The model under review builds one solid part; all positions refer to its coordinate system, in mm. A direction names the side the tool comes from. Round coordinates to 2 decimals unless told otherwise and drop trailing zeros. Order: outer loops, then holes, each group sorted by start corner. A loop starts at its lowest first (then second) coordinate and runs counter-clockwise, first axis right, second up.
1) Clearance check with flat-ended pins moving along their axes: P1, Ø8, axis at x = -67, z = -3.5, coming from the -Y side; P2, Ø1.5, axis at x = -6, z = -21.5, coming from the +Y side; P3, Ø9, axis at y = 243, z = -5.5, coming from the +X side; P4, Ø8, axis at x = 0, y = 260, coming from the +Z side. State where each tip first meets the part, or that it passes through.
2) To check wall thickness, follow L1, parallel to X at y = 260, z = -0.5; L2, parallel to X at y = 53, z = 0; L3, parallel to Y at x = 0, z = -8. State the ranges of each line that lie inside material, in increasing order.
3) Consider section C-C (x = 18). Give the boundary of the cut face in (y, z).
4) Consider section B-B (z = 0). Give the boundary of the cut face in (x, y), then the cut area to 3 significant figures.
5) Machinability: for faces 1 (the face through (10.382, 101.4, 19.961)), 2 (the face through (15, 245, 0)), 3 (the face through (-50, 100, 0)), which of the approach directions +Z, -Z, +X, -X, +Y, -Y give a long, thin tool a straight path to every point of the face, cutting with its end or side? Answer none if there is none.
6) Consider section D-D (y = 211). Give the boundary of the cut face in (x, z).
7) Consider section A-A (y = 162.5). Give the boundary of the cut face in (x, z), then the cut area to 3 significant figures.
8) Mouldability with a two-part tool opening along Z and no side actions: class faces 4 (the face through (-1.172, 101.4, -8.923)), 5 (the face through (0, 200, 0)), 6 (the face through (0, 253, 15)), 7 (the face through (-0.651, 264.957, -0.21)) as pulls with the +Z half, pulls with the -Z half, needs draft (parallel to the pull), parting line crosses it, or undercut.
from build123d import *

# Parameters (mm, degrees)
ESBO_O1_W                = 13.5
ESBO_O1_H                = 200
RESSALTO_EXTRUS_O1_DEPTH = 30
ESBO_O3_W                = 25
ESBO_O3_H                = 100
ESBO_O4_R                = 5
RESSALTO_EXTRUS_O2_DEPTH = 15


with BuildPart() as part:
    # Esboço1 → Revolução1 (revolve)
    with BuildSketch(Plane.XY):
        with Locations((15.75, 100)):
            Rectangle(ESBO_O1_W, ESBO_O1_H)
    revolve(axis=Axis((0, 0, 0), (0, 1, 0)))

    # Esboço2 → Ressalto-extrusão1 (add)
    with BuildSketch(Plane(origin=(0, 200, 0), x_dir=(1, 0, 0), z_dir=(0, 1, 0))):
        with BuildLine():
            Line((0, -30), (-50, -30))
            ThreePointArc((-50, -30), (-80, 0), (-50, 30))
            Line((-50, 30), (0, 30))
            ThreePointArc((0, 30), (30, 0), (0, -30))
        make_face()
    extrude(amount=RESSALTO_EXTRUS_O1_DEPTH)

    # Esboço3 → Revolução2 (revolve)
    with BuildSketch(Plane.XY):
        with Locations((-37.5, 150)):
            Rectangle(ESBO_O3_W, ESBO_O3_H)
    revolve(axis=Axis((-50, 200, 0), (0, -1, 0)))

    # Esboço4 → Ressalto-extrusão2 (add, symmetric)
    with BuildSketch(Plane.XY):
        with BuildLine():
            Line((15, 230), (15, 260))
            ThreePointArc((15, 260), (0, 275), (-15, 260))
            Line((-15, 260), (-15, 230))
            Line((-15, 230), (15, 230))
        make_face()
        with Locations((0, 260)):
            Circle(ESBO_O4_R, mode=Mode.SUBTRACT)
    extrude(amount=RESSALTO_EXTRUS_O2_DEPTH, both=True)


solid = part.part
Answer below:
1. P1: stops at y = 100
1. P2: stops at y = 230
1. P3: stops at x = 15
1. P4: passes through
2. L1: x = -15 to -5, 5 to 15
2. L2: x = -22.5 to -9, 9 to 22.5
2. L3: y = 200 to 255, 265 to 275
3. outline: (0, -13.5) - (200, -13.5) - (200, -24) - (230, -24) - (230, 24) - (200, 24) - (200, 13.5) - (0, 13.5) - close
4. outline: (-80, 200) - (-75, 200) - (-75, 100) - (-25, 100) - (-25, 200) - (-22.5, 200) - (-22.5, 0) - (-9, 0) - (-9, 200) - (9, 200) - (9, 0) - (22.5, 0) - (22.5, 200) - (30, 200) - (30, 230) - (15, 230) - (15, 260) arc R15 ccw to (-15, 260) - (-15, 230) - (-80, 230) - close; hole circle Ø10 at (0, 260)
4. area: 14,900 mm2
5. face 1: -Y
5. face 2: +Z, -Z, +X, +Y
5. face 3: +Z, -Z, -X, -Y
6. outline: (-50, -30) - (0, -30) arc R30 ccw to (0, 30) - (-50, 30) arc R30 ccw to start
7. outline: circle Ø50 at (-50, 0); circle Ø45 at (0, 0); hole circle Ø18 at (0, 0)
7. area: 3,300 mm2
8. face 4: undercut
8. face 5: undercut
8. face 6: pulls with the +Z half
8. face 7: needs draft
